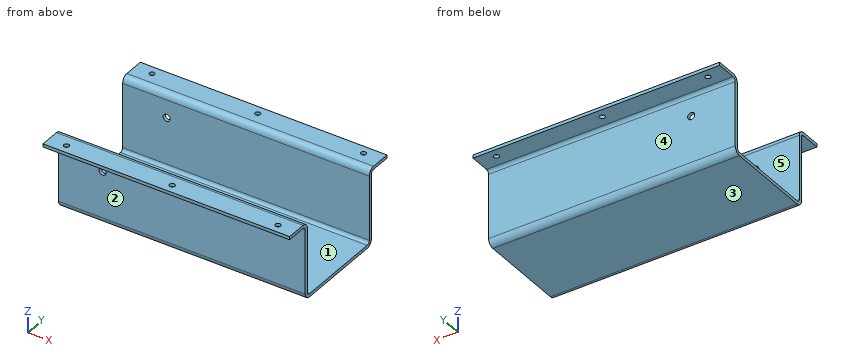
from build123d import *

# Parameters (mm, degrees)
BASE_FLANGE1_DEPTH           = 88.9
F_25_0_1495_DIAMETER_HOLE1_D = 3.7973
F_7_0_201_DIAMETER_HOLE1_D   = 5.1054


# Sheet-metal steps are written as plain solids
with BuildPart() as part:
    # Sketch1 → Base-Flange1 (new, symmetric)
    with BuildSketch(Plane.YZ):
        with BuildLine():
            Line((-52.3875, 26.67), (-37.9095, 26.67))
            ThreePointArc((-37.9095, 26.67), (-34.676607796, 25.330892204), (-33.3375, 22.098))
            Line((-33.3375, 22.098), (-33.3375, -24.384))
            ThreePointArc((-33.3375, -24.384), (-32.667946102, -26.000446102), (-31.0515, -26.67))
            Line((-31.0515, -26.67), (31.0515, -26.67))
            ThreePointArc((31.0515, -26.67), (32.667946102, -26.000446102), (33.3375, -24.384))
            Line((33.3375, -24.384), (33.3375, 22.098))
            ThreePointArc((33.3375, 22.098), (34.676607796, 25.330892204), (37.9095, 26.67))
            Line((37.9095, 26.67), (52.3875, 26.67))
            Line((52.3875, 26.67), (52.3875, 24.384))
            Line((52.3875, 24.384), (37.9095, 24.384))
            ThreePointArc((37.9095, 24.384), (36.293053898, 23.714446102), (35.6235, 22.098))
            Line((35.6235, 22.098), (35.6235, -24.384))
            ThreePointArc((35.6235, -24.384), (34.284392204, -27.616892204), (31.0515, -28.956))
            Line((31.0515, -28.956), (-31.0515, -28.956))
            ThreePointArc((-31.0515, -28.956), (-34.284392204, -27.616892204), (-35.6235, -24.384))
            Line((-35.6235, -24.384), (-35.6235, 22.098))
            ThreePointArc((-35.6235, 22.098), (-36.293053898, 23.714446102), (-37.9095, 24.384))
            Line((-37.9095, 24.384), (-52.3875, 24.384))
            Line((-52.3875, 24.384), (-52.3875, 26.67))
        make_face()
    extrude(amount=BASE_FLANGE1_DEPTH, both=True)

    # #25 (0.1495) Diameter Hole1 (through all)
    with Locations(Plane.XY.offset(26.67)):
        with Locations((-76.2, 46.0375), (0, 46.0375), (76.2, 46.0375), (76.2, -46.0375), (0, -46.0375), (-76.2, -46.0375)):
            Hole(F_25_0_1495_DIAMETER_HOLE1_D / 2)

    # #7 (0.201) Diameter Hole1 (through all)
    with Locations(Plane.XZ.offset(35.6235)):
        with Locations((-57.15, 9.144)):
            Hole(F_7_0_201_DIAMETER_HOLE1_D / 2)


solid = part.part
Input: part model. Units: mm. Frame: model coordinates. Face numbers are marked on the shaded views. A direction names the side the tool comes from. Round coordinates to 2 decimals unless told otherwise and drop trailing zeros. Loops run counter-clockwise (first coordinate to the right, second up) from the corner with the lowest first, then second, coordinate; pieces in that order, holes last. Notation, with made-up numbers: M 16.25,48.25 L 43.25,48.25 A4 ccw 43.25,55.25 Z; hole C 43,-26.75 d6. An arc over 180 degrees is marked long. Answer as CSV lines item,"result". Start each with the question number.
(1) Section B-B, the plane z = 16. Output: boundary loops of the cut face in (x, y).
(2) First-contact query: pin 1 (14 mm diameter, centred on x = -26, z = 6.5, fed in from -Y); pin 2 (12 mm diameter, centred on x = 53, z = -23.5, fed in from +Y); pin 3 (6 mm diameter, centred on x = 5, y = -10.5, fed in from +Z). Flat tips, straight axial feed; report the tip coordinate or a pass-through.
(3) Draft query along Y for the marked faces 3, 4 and 5. Return one class per face: released by +Y, released by -Y, zero draft, split by the parting line, or undercut.
(4) Section D-D, the plane x = -57.15. Output: boundary loops of the cut face in (y, z), plus the area to 3 significant figures.
(5) Reachability of the marked faces 1 and 2 from +Z, -Z, +X, -X, +Y, -Y: full face, straight path, thin tool, end or side. Return the list, or none.
(6) Section A-A, the plane x = 76.2. Output: boundary loops of the cut face in (y, z).
(7) Line query: line 1 (Y direction, x = -29, z = 4); line 2 (Y direction, x = 76.2, z = 25.5); line 3 (Y direction, x = -76.2, z = 25.4). Output: solid intervals per line, ascending. Write a range as [from, to].
(8) Section C-C, the plane x = 33.5. Output: boundary loops of the cut face in (y, z).
Values found:
1,outline,"M -88.9,-35.62 L 88.9,-35.62 L 88.9,-33.34 L -88.9,-33.34 Z; M -88.9,33.34 L 88.9,33.34 L 88.9,35.62 L -88.9,35.62 Z"
2,pin 1,"stops at y = -35.62"
2,pin 2,"stops at y = 35.62"
2,pin 3,"stops at z = -26.67"
3,face 3,"zero draft"
3,face 4,"released by +Y"
3,face 5,"undercut"
4,outline,"M -52.39,24.38 L -37.91,24.38 A2.29 cw -35.62,22.1 L -35.62,11.7 L -33.34,11.7 L -33.34,22.1 A4.57 ccw -37.91,26.67 L -52.39,26.67 Z; M -35.62,-24.38 A4.57 ccw -31.05,-28.96 L 31.05,-28.96 A4.57 ccw 35.62,-24.38 L 35.62,6.59 L 33.34,6.59 L 33.34,-24.38 A2.29 cw 31.05,-26.67 L -31.05,-26.67 A2.29 cw -33.34,-24.38 L -33.34,6.59 L -35.62,6.59 Z; M 33.34,11.7 L 35.62,11.7 L 35.62,22.1 A2.29 cw 37.91,24.38 L 52.39,24.38 L 52.39,26.67 L 37.91,26.67 A4.57 ccw 33.34,22.1 Z"
4,area,"447 mm²"
5,face 1,"+Z, +X, -X"
5,face 2,"-Z, +X, -X, -Y"
6,outline,"M -52.39,24.38 L -47.94,24.38 L -47.94,26.67 L -52.39,26.67 Z; M -44.14,24.38 L -37.91,24.38 A2.29 cw -35.62,22.1 L -35.62,-24.38 A4.57 ccw -31.05,-28.96 L 31.05,-28.96 A4.57 ccw 35.62,-24.38 L 35.62,22.1 A2.29 cw 37.91,24.38 L 44.14,24.38 L 44.14,26.67 L 37.91,26.67 A4.57 ccw 33.34,22.1 L 33.34,-24.38 A2.29 cw 31.05,-26.67 L -31.05,-26.67 A2.29 cw -33.34,-24.38 L -33.34,22.1 A4.57 ccw -37.91,26.67 L -44.14,26.67 Z; M 47.94,24.38 L 52.39,24.38 L 52.39,26.67 L 47.94,26.67 Z"
7,line 1,"y = [-35.62, -33.34], [33.34, 35.62]"
7,line 2,"y = [-52.39, -47.94], [-44.14, -34.86], [34.86, 44.14], [47.94, 52.39]"
7,line 3,"y = [-52.39, -47.94], [-44.14, -34.75], [34.75, 44.14], [47.94, 52.39]"
8,outline,"M -52.39,24.38 L -37.91,24.38 A2.29 cw -35.62,22.1 L -35.62,-24.38 A4.57 ccw -31.05,-28.96 L 31.05,-28.96 A4.57 ccw 35.62,-24.38 L 35.62,22.1 A2.29 cw 37.91,24.38 L 52.39,24.38 L 52.39,26.67 L 37.91,26.67 A4.57 ccw 33.34,22.1 L 33.34,-24.38 A2.29 cw 31.05,-26.67 L -31.05,-26.67 A2.29 cw -33.34,-24.38 L -33.34,22.1 A4.57 ccw -37.91,26.67 L -52.39,26.67 Z"
